from build123d import *

# Parameters (mm, degrees)
GRAY_HOUSING_PERIMETER_RETENTION_START = 11
SKETCH_1_W                             = 51
SKETCH_1_H                             = 22.4
SKETCH_1_W_2                           = 48.4
SKETCH_1_H_2                           = 19
GRAY_HOUSING_PERIMETER_RETENTION_DEPTH = 7
GRAY_LOWER_EDGE_RETAINING_LIPS_START   = 9.5
SKETCH_2_W                             = 51
SKETCH_2_H                             = 2.8
GRAY_LOWER_EDGE_RETAINING_LIPS_DEPTH   = 1.5
GRAY_MOUNTING_ENDS_TO_DECK_START       = 12
SKETCH_5_W                             = 7.5
SKETCH_5_H                             = 10
GRAY_MOUNTING_ENDS_TO_DECK_DEPTH       = 10
GRAY_M3_MOUNTS_START                   = 23
SKETCH_6_R                             = 1.7
GRAY_M3_MOUNTS_DEPTH                   = 12


with BuildPart() as part:
    # 草图1 → Gray_housing_perimeter_retention (new body)
    with BuildSketch(Plane.XY.offset(GRAY_HOUSING_PERIMETER_RETENTION_START)):
        Rectangle(SKETCH_1_W, SKETCH_1_H)
        Rectangle(SKETCH_1_W_2, SKETCH_1_H_2, mode=Mode.SUBTRACT)
    extrude(amount=GRAY_HOUSING_PERIMETER_RETENTION_DEPTH)

    # 草图2 → Gray_lower_edge_retaining_lips (add)
    with BuildSketch(Plane.XY.offset(GRAY_LOWER_EDGE_RETAINING_LIPS_START)):
        with Locations((0, -9.8)):
            Rectangle(SKETCH_2_W, SKETCH_2_H)
        with Locations((0, 9.8)):
            Rectangle(SKETCH_2_W, SKETCH_2_H)
    extrude(amount=GRAY_LOWER_EDGE_RETAINING_LIPS_DEPTH)

    # 草图5 → Gray_mounting_ends_to_deck (add)
    with BuildSketch(Plane.XY.offset(GRAY_MOUNTING_ENDS_TO_DECK_START)):
        with Locations((-28.25, 0)):
            Rectangle(SKETCH_5_W, SKETCH_5_H)
        with Locations((28.25, 0)):
            Rectangle(SKETCH_5_W, SKETCH_5_H)
    extrude(amount=GRAY_MOUNTING_ENDS_TO_DECK_DEPTH)

    # 草图6 → Gray_M3_mounts (cut)
    with BuildSketch(Plane.XY.offset(GRAY_M3_MOUNTS_START)):
        with Locations(Location((-28.5, 0, 0), (0, 0, 180))):
            Circle(SKETCH_6_R)
        with Locations(Location((28.5, 0, 0), (0, 0, 180))):
            Circle(SKETCH_6_R)
    extrude(amount=-GRAY_M3_MOUNTS_DEPTH, mode=Mode.SUBTRACT)


solid = part.part
Can you work these out from the model? Positions are in its coordinate system, mm. A direction names the side the tool comes from. Give positions to 0.01 mm unless a question says otherwise; leave off trailing zeros. Write each loop counter-clockwise with the first axis right and the second up, starting at its lowest first coordinate (ties: lowest second). Pieces come first, ordered by that corner, then holes. Notation, with made-up numbers: M 86.25,21.25 L 140.25,21.25 A6 cw 140.25,32.25 Z; hole C 66,-30 d6. An arc over 180 degrees is marked long. Answer in a Markdown table with one row per item. Add a question column.
Item 1: Imagine slicing it at D-D, the plane y = -6.25. Write out the boundary of the cut face in (x, z).
Item 2: Imagine slicing it at B-B, the plane y = 0. Write out the boundary of the cut face in (x, z), plus the area to 3 significant figures.
Item 3: We'd pull the mould along Y, two halves only. Please class faces 1 (the cylindrical face through (26.93, 0.65, 17.07)), 2 (the flat face through (2, 10, 18)), 3 (the flat face through (0, 11.2, 14)): released by +Y, released by -Y, zero draft, split by the parting line, or undercut.
Item 4: Imagine slicing it at A-A, the plane x = 19.5. Write out the boundary of the cut face in (y, z).
Item 5: Imagine slicing it at C-C, the plane z = 14. Write out the boundary of the cut face in (x, y), plus the area to 3 significant figures.
Item 6: Please list where these lines run through material, in increasing order: L1, parallel to Y at x = 10, z = 16; L2, parallel to X at y = 6.25, z = 11.5; L3, parallel to X at y = -3, z = 17.5.
Item 7: For pin 1 Ø7 at (x, y) = (-28.5, 1) entering from -Z; pin 2 Ø8 at (x, y) = (-7.5, -7.5) entering from -Z; pin 3 Ø3 at (x, y) = (29, -2) entering from -Z; pin 4 Ø6 at (x, z) = (-29, 14.5) entering from +Y, each with a flat end and sliding along its axis, tell me the tip position at first contact or that it passes through.
Item 8: On a 3-axis mill with a long thin cutter (end or side, diameter ignored), from which of +Z, -Z, +X, -X, +Y, -Y can I reach the whole of each face in a straight line? I mean faces 4 (the flat face through (-30.2, -1, 12)), 5 (the flat face through (30.1, 1.2, 12)), 6 (the flat face through (-25, 0, 11)), 7 (the flat face through (24.5, 0, 20)). Say none if no direction works.
Evaluation:
| question | item | result |
|---|---|---|
| 1 | outline | M -25.5,11 L -24.2,11 L -24.2,18 L -25.5,18 Z; M 24.2,11 L 25.5,11 L 25.5,18 L 24.2,18 Z |
| 2 | outline | M -32,12 L -30.2,12 L -30.2,22 L -32,22 Z; M -26.8,12 L -25.5,12 L -25.5,11 L -24.2,11 L -24.2,18 L -24.5,18 L -24.5,22 L -26.8,22 Z; M 24.2,11 L 25.5,11 L 25.5,12 L 26.8,12 L 26.8,22 L 24.5,22 L 24.5,18 L 24.2,18 Z; M 30.2,12 L 32,12 L 32,22 L 30.2,22 Z |
| 2 | area | 88.2 mm² |
| 3 | face 1 | undercut |
| 3 | face 2 | zero draft |
| 3 | face 3 | released by +Y |
| 4 | outline | M -11.2,9.5 L -8.4,9.5 L -8.4,11 L -9.5,11 L -9.5,18 L -11.2,18 Z; M 8.4,9.5 L 11.2,9.5 L 11.2,18 L 9.5,18 L 9.5,11 L 8.4,11 Z |
| 5 | outline | M -32,-5 L -25.5,-5 L -25.5,-11.2 L 25.5,-11.2 L 25.5,-5 L 32,-5 L 32,5 L 25.5,5 L 25.5,11.2 L -25.5,11.2 L -25.5,5 L -32,5 Z; hole C -28.5,0 d3.4; hole M -24.2,-9.5 L 24.2,-9.5 L 24.2,9.5 L -24.2,9.5 Z; hole C 28.5,0 d3.4 |
| 5 | area | 335 mm² |
| 6 | L1 | y = -11.2 to -9.5, 9.5 to 11.2 |
| 6 | L2 | x = -25.5 to -24.2, 24.2 to 25.5 |
| 6 | L3 | x = -32 to -24.2, 24.2 to 32 |
| 7 | pin 1 | stops at z = 11 |
| 7 | pin 2 | stops at z = 9.5 |
| 7 | pin 3 | stops at z = 12 |
| 7 | pin 4 | stops at y = 5 |
| 8 | face 4 | -Z, -X, +Y, -Y |
| 8 | face 5 | -Z, +X, +Y, -Y |
| 8 | face 6 | -Z, +X, -X |
| 8 | face 7 | +Z, +Y, -Y |
